The model under review builds one solid part; all positions refer to its coordinate system, in mm. A direction names the side the tool comes from. Give positions to 0.01 mm unless a question says otherwise; leave off trailing zeros. Order: outer loops, then holes, each group sorted by start corner. A loop starts at its lowest first (then second) coordinate and runs counter-clockwise, first axis right, second up. Notation, with made-up numbers: (33, -27.5) -> (53, -27.5) arc R33 ccw to (53, 11.5) -> close; hole circle Ø2 at (6.25, 79). An arc over 180 degrees is marked (long way). Use one line per item in the form item = value.
Autodesk Inventor part; units mm, degrees
ref_plane "우측면도" through (0, 0, 0) normal (1, 0, 0) x (0, 1, 0)
ref_plane "평면도" through (0, 0, 0) normal (0, 1, 0) x (-1, 0, 0)
ref_plane "정면도" through (0, 0, 0) normal (0, 0, 1) x (1, 0, 0)
sketch "스케치1" plane through (0, 0, 0) normal (0, 1, 0) x (-1, 0, 0)
  line L0 (-37, 35) -> (37, 35)
  line L1 (37, 35) -> (37, -35)
  line L2 (37, -35) -> (-37, -35)
  line L3 (-37, -35) -> (-37, 35)
  line L4 (-37, 35) -> (37, -35) construction
  line L5 (37, 35) -> (-37, -35) construction
  line L6 (37, -14) -> (37, -2)
  line L7 (-37, -14) -> (-37, -2)
  line L8 (28.9, 13.6) -> (31.1, 13.6)
  line L9 (31.1, 13.6) -> (31.1, 8.4)
  line L10 (31.1, 8.4) -> (28.9, 8.4)
  line L11 (28.9, 8.4) -> (28.9, 13.6)
  line L12 (28.9, 13.6) -> (31.1, 8.4) construction
  line L13 (31.1, 13.6) -> (28.9, 8.4) construction
  line L14 (-31.1, 13.6) -> (-28.9, 13.6)
  line L15 (-28.9, 13.6) -> (-28.9, 8.4)
  line L16 (-28.9, 8.4) -> (-31.1, 8.4)
  line L17 (-31.1, 8.4) -> (-31.1, 13.6)
  line L18 (-31.1, 13.6) -> (-28.9, 8.4) construction
  line L19 (-28.9, 13.6) -> (-31.1, 8.4) construction
  line L20 (-31.1, -8.4) -> (-28.9, -8.4)
  line L21 (-28.9, -8.4) -> (-28.9, -13.6)
  line L22 (-28.9, -13.6) -> (-31.1, -13.6)
  line L23 (-31.1, -13.6) -> (-31.1, -8.4)
  line L24 (-31.1, -8.4) -> (-28.9, -13.6) construction
  line L25 (-28.9, -8.4) -> (-31.1, -13.6) construction
  line L26 (31.1, -8.4) -> (28.9, -8.4)
  line L27 (28.9, -8.4) -> (28.9, -13.6)
  line L28 (28.9, -13.6) -> (31.1, -13.6)
  line L29 (31.1, -13.6) -> (31.1, -8.4)
  line L30 (31.1, -8.4) -> (28.9, -13.6) construction
  line L31 (28.9, -8.4) -> (31.1, -13.6) construction
  line L32 (37, 6) -> (43, 6)
  line L33 (43, 6) -> (43, -6)
  line L34 (43, -6) -> (37, -6)
  line L35 (37, -6) -> (37, 6)
  line L36 (-37, 6) -> (-43, 6)
  line L37 (-43, 6) -> (-43, -6)
  line L38 (-43, -6) -> (-37, -6)
  line L39 (-37, -6) -> (-37, 6)
  circle A0 centre (20.8, 30.8) radius 1.6
  circle A1 centre (20.8, -30.8) radius 1.6
  circle A2 centre (-20.8, 30.8) radius 1.6
  circle A3 centre (-20.8, -30.8) radius 1.6
  circle A4 centre (28.8, 30.8) radius 1.35
  circle A5 centre (28.8, -30.8) radius 1.35
  circle A6 centre (-28.8, 30.8) radius 1.35
  circle A7 centre (-28.8, -30.8) radius 1.35
  point P0 (0, 0)
  point P1 (30, 11)
  point P2 (-30, 11)
  point P3 (-30, -11)
  point P4 (30, -11)
  dimension "d0" = 74
  dimension "d1" = 70
  dimension "d6" = 2.2
  dimension "d7" = 5.2
  dimension "d8" = 2.2
  dimension "d9" = 5.2
  dimension "d10" = 2.2
  dimension "d11" = 5.2
  dimension "d12" = 2.2
  dimension "d13" = 5.2
  dimension "d14" = 6
  dimension "d15" = 12
  dimension "d16" = 6
  dimension "d17" = 12
  dimension "d18" = 3.2
  dimension "d19" = 4.2
  dimension "d20" = 3.2
  dimension "d21" = 3.2
  dimension "d22" = 3.2
  dimension "d23" = 2.7
  dimension "d24" = 2.7
  dimension "d25" = 2.7
  dimension "d26" = 2.7
extrude "돌출1" add sketch "스케치1" along normal blind 6
sketch "스케치2" plane through (37, 0, 35) normal (1, 0, 0) x (0, 0, -1)
  circle A0 centre (46, 3) radius 1.35
  circle A1 centre (24, 3) radius 1.35
  point P0 (35, 0)
  dimension "d29" = 2.7
  dimension "d30" = 2.7
extrude "돌출2" cut sketch "스케치2" against normal blind 100
sketch "스케치3" plane through (-37, 0, 35) normal (0, 0, 1) x (1, 0, 0)
  line L0 (0, 0) -> (74, 0)
  line L1 (74, 0) -> (74, 6)
  line L2 (74, 6) -> (0, 6)
  line L3 (0, 6) -> (0, 0)
  point P0 (37, 0)
  dimension "d33" = 74
  dimension "d34" = 6
extrude "돌출3" add sketch "스케치3" along normal blind 10
sketch "스케치4" plane through (0, 6, 0) normal (0, 1, 0) x (1, 0, 0)
  circle A0 centre (20, -40) radius 1.35
  circle A1 centre (-20, -40) radius 1.35
  line L0 (-6.05, -43.05) -> (6.05, -43.05)
  line L1 (6.05, -43.05) -> (6.05, -36.95)
  line L2 (6.05, -36.95) -> (-6.05, -36.95)
  line L3 (-6.05, -36.95) -> (-6.05, -43.05)
  line L4 (-6.05, -43.05) -> (6.05, -36.95) construction
  line L5 (6.05, -43.05) -> (-6.05, -36.95) construction
  point P0 (0, 0)
  point P1 (0, -40)
  dimension "d37" = 2.7
  dimension "d38" = 2.7
  dimension "d39" = 12.1
  dimension "d40" = 6.1
extrude "돌출4" cut sketch "스케치4" against normal blind 10
sketch "스케치5" plane through (0, 6, 0) normal (0, 1, 0) x (1, 0, 0)
  circle A0 centre (0, 0) radius 12.5
  dimension "d43" = 25
extrude "돌출5" cut sketch "스케치5" against normal blind 10
sketch "스케치6" plane through (0, 6, 0) normal (0, 1, 0) x (1, 0, 0)
  circle A0 centre (0, 0) radius 12.5
  circle A1 centre (20, -40) radius 1.35
  circle A2 centre (-20, -40) radius 1.35
  line L0 (-6.05, -36.95) -> (6.05, -36.95)
  line L1 (6.05, -36.95) -> (6.05, -43.05)
  line L2 (6.05, -43.05) -> (-6.05, -43.05)
  line L3 (-6.05, -43.05) -> (-6.05, -36.95)
  line L4 (37, -6) -> (37, -45)
  line L5 (37, -6) -> (43, -6)
  line L6 (43, -6) -> (43, 6)
  line L7 (43, 6) -> (37, 6)
  line L8 (37, 6) -> (37, 35)
  line L9 (37, 35) -> (-37, 35)
  line L10 (-37, 35) -> (-37, 6)
  line L11 (-37, 6) -> (-43, 6)
  line L12 (-43, 6) -> (-43, -6)
  line L13 (-43, -6) -> (-37, -6)
  line L14 (-37, -6) -> (-37, -45)
  line L15 (37, -45) -> (-37, -45)
  circle A3 centre (28.8, 30.8) radius 1.35
  circle A4 centre (-28.8, 30.8) radius 1.35
  circle A5 centre (-28.8, -30.8) radius 1.35
  circle A6 centre (20.8, 30.8) radius 1.6
  circle A7 centre (20.8, -30.8) radius 1.6
  circle A8 centre (-20.8, 30.8) radius 1.6
  circle A9 centre (-20.8, -30.8) radius 1.6
  circle A10 centre (28.8, -30.8) radius 1.35
  line L16 (-31.1, 8.4) -> (-31.1, 13.6)
  line L17 (-31.1, 13.6) -> (-28.9, 13.6)
  line L18 (-28.9, 13.6) -> (-28.9, 8.4)
  line L19 (-28.9, 8.4) -> (-31.1, 8.4)
  line L20 (31.1, 8.4) -> (28.9, 8.4)
  line L21 (28.9, 8.4) -> (28.9, 13.6)
  line L22 (28.9, 13.6) -> (31.1, 13.6)
  line L23 (31.1, 13.6) -> (31.1, 8.4)
  line L24 (31.1, -13.6) -> (28.9, -13.6)
  line L25 (28.9, -13.6) -> (28.9, -8.4)
  line L26 (28.9, -8.4) -> (31.1, -8.4)
  line L27 (31.1, -8.4) -> (31.1, -13.6)
  line L28 (-28.9, -13.6) -> (-31.1, -13.6)
  line L29 (-31.1, -13.6) -> (-31.1, -8.4)
  line L30 (-31.1, -8.4) -> (-28.9, -8.4)
  line L31 (-28.9, -8.4) -> (-28.9, -13.6)
  circle A11 centre (-6.05, -36.95) radius 1
  circle A12 centre (-6.05, -43.05) radius 1
  circle A13 centre (6.05, -36.95) radius 1
  circle A14 centre (6.05, -43.05) radius 1
  circle A15 centre (-37, -6) radius 1
  circle A16 centre (-37, 6) radius 1
  circle A17 centre (37, -6) radius 1
  circle A18 centre (37, 6) radius 1
  point P0 (38, -6)
  point P1 (37, -7)
  point P2 (37, 7)
  point P3 (38, 6)
  point P4 (-37, 7)
  point P5 (-38, 6)
  point P6 (-37, -7)
  point P7 (-38, -6)
  dimension "d46" = 2
  dimension "d47" = 2
  dimension "d48" = 2
  dimension "d49" = 2
  dimension "d50" = 2
  dimension "d51" = 2
  dimension "d52" = 2
  dimension "d53" = 2
extrude "돌출6" cut sketch "스케치6" against normal through all contours L3 A11 L0 | L0 A11 L3 | A13 L1 L0 | L0 L1 A13 | A12 L2 L3 | L3 L2 A12 | A14 L2 L1 | L1 L2 A14 | L4 A17 L5 | L14 L13 A15 | A18 L8 L7 | L11 L10 A16 picked at (36.9727, -5.339) picked at (-37.657, -5.9202) picked at (36.9727, 5.339) picked at (-36.343, 5.9202)
properties part number "under the head" material "PMMA 플라스틱"
1. Add section C-C on z = -11. Count the separate pieces of the cut face and the enclosed holes in it, then the cut area to 3 significant figures.
Values:
separate_pieces = 8
enclosed_holes = 0
area = 190 mm^2
2. Add section D-D on z = 18.5. Give the boundary of the cut face in (x, y).
Values:
outline = (-37, 0) -> (37, 0) -> (37, 6) -> (-37, 6) -> close
3. For L1, parallel to Z at x = 22.5, y = 3; L2, parallel to X at y = 3.75, z = -13; L3, parallel to Z at x = 31, y = 3.5, list the stretches that pass through material, from the lowest coordinate up.
Values:
L1 = -35 to -12.35, -9.65 to 9.65, 12.35 to 45
L2 = -37 to -31.1, -28.9 to 28.9, 31.1 to 37
L3 = -35 to -13.6, -8.4 to 8.4, 13.6 to 45
4. For pin 1 Ø1.8 at (y, z) = (3, 24) entering from +X; pin 2 Ø2.5 at (y, z) = (3.5, -12) entering from -X; pin 3 Ø1.9 at (x, z) = (-20.8, 30.8) entering from +Y, all flat-tipped, find the tip position at first contact; note any pin that passes through.
Values:
pin_1 = 37
pin_2 = -37
pin_3 = through
5. The part is to be moulded in two halves that separate along Z. For faces 1 (the face through (-41, 3, -6)), 2 (the face through (-1, 3, 45)), 3 (the face through (-19.62, 2.96, -31.88)), say which applies: +Z half, -Z half, draft (parallel to the pull), parting line (faces both ways), or undercut.
Values:
face_1 = -Z half
face_2 = +Z half
face_3 = undercut
6. Tool access review of faces 4 (the face through (-34.009, 2.483, -12.247)), 5 (the face through (-40, 3, 6)), 6 (the face through (28.9, 1.6, -10.4)): name each direction out of +Z, -Z, +X, -X, +Y, -Y from which nothing blocks a thin tool from reaching the whole face with its end or side.
Values:
face_4 = +X, -X
face_5 = +Z, -X, +Y, -Y
face_6 = +Y, -Y
7. Add section B-B on z = 40. Give the boundary of the cut face in (x, y).
Values:
outline = (-37, 0) -> (-21.35, 0) -> (-21.35, 6) -> (-37, 6) -> close; (-18.65, 0) -> (-6.05, 0) -> (-6.05, 6) -> (-18.65, 6) -> close; (6.05, 0) -> (18.65, 0) -> (18.65, 6) -> (6.05, 6) -> close; (21.35, 0) -> (37, 0) -> (37, 6) -> (21.35, 6) -> close
8. Add section A-A on z = 30.8. Give the boundary of the cut face in (x, y).
Values:
outline = (-37, 0) -> (-30.15, 0) -> (-30.15, 6) -> (-37, 6) -> close; (-27.45, 0) -> (-22.4, 0) -> (-22.4, 6) -> (-27.45, 6) -> close; (-19.2, 0) -> (19.2, 0) -> (19.2, 6) -> (-19.2, 6) -> close; (22.4, 0) -> (27.45, 0) -> (27.45, 6) -> (22.4, 6) -> close; (30.15, 0) -> (37, 0) -> (37, 6) -> (30.15, 6) -> close
